Part model, mm, in its own coordinate system. Face numbers are marked on the shaded views. Round coordinates to 2 decimals unless told otherwise and drop trailing zeros. Write each loop counter-clockwise with the first axis right and the second up, starting at its lowest first coordinate (ties: lowest second). Pieces come first, ordered by that corner, then holes.
1) Saw through at B-B on x = 2. Write the cut outline in (y, z), and give its area (3 significant figures).
2) Flat gauge pins, fed straight in: pin 1 (1.5 mm diameter, centred on x = 0.5, z = 0, fed in from +Y); pin 2 (2 mm diameter, centred on x = 1, y = 23.5, fed in from -Z); pin 3 (3 mm diameter, centred on y = 21.5, z = -0.5, fed in from +X). Where does each tip first touch, or does it go through?
3) Saw through at D-D on y = 16.75. Write the cut outline in (x, z), and give its area (3 significant figures).
4) Saw through at C-C on z = 1.9. Write the cut outline in (x, y), and give its area (3 significant figures).
5) Pull direction Z, two halves, no side cores. Call the marked faces 1, 2 and 3: +Z half, -Z half, draft (parallel to the pull), parting line (faces both ways), or undercut.
6) Saw through at A-A on y = 25.5. Write the cut outline in (x, z), and give its area (3 significant figures).
7) Drill centre lines: L1, parallel to Y at x = -1.85, z = -1.4; L2, parallel to Z at x = -0.3, y = 26; L3, parallel to Z at x = 0.5, y = 26. Where is each one in solid material? Low to high.
```python
from build123d import *

# Parameters (mm, degrees)
SKETCH1_R                                           = 2.5
BOSS_EXTRUDE1_DEPTH                                 = 0.5
SKETCH2_R                                           = 2.25
BOSS_EXTRUDE2_DEPTH                                 = 27.7
CSK_FOR_M2_COUNTERSUNK_FLAT_HEAD_SCREW1_D           = 2.2
CSK_FOR_M2_COUNTERSUNK_FLAT_HEAD_SCREW1_DEPTH       = 9.339053319
CSK_FOR_M2_COUNTERSUNK_FLAT_HEAD_SCREW1_CSINK_D     = 3
CSK_FOR_M2_COUNTERSUNK_FLAT_HEAD_SCREW1_CSINK_ANGLE = 90
CSK_FOR_M2_COUNTERSUNK_FLAT_HEAD_SCREW1_TIP         = 0.660946681


with BuildPart() as part:
    # Sketch1 → Boss-Extrude1 (new body)
    with BuildSketch(Plane(origin=(0, 0, 0), x_dir=(1, 0, 0), z_dir=(0, 1, 0))):
        with Locations(Location((0, 0, 0), (0, 0, 270))):
            Circle(SKETCH1_R)
    extrude(amount=BOSS_EXTRUDE1_DEPTH)

    # Sketch2 → Boss-Extrude2 (add)
    with BuildSketch(Plane(origin=(0, 0.5, 0), x_dir=(1, 0, 0), z_dir=(0, 1, 0))):
        with Locations(Location((0, 0, 0), (0, 0, 270))):
            Circle(SKETCH2_R)
    extrude(amount=BOSS_EXTRUDE2_DEPTH)

    # CSK for M2 Countersunk Flat Head Screw1
    with Locations(Plane(origin=(0, 28.2, 0), x_dir=(1, 0, 0), z_dir=(0, 1, 0))):
        with Locations((0, 0)):
            CounterSinkHole(CSK_FOR_M2_COUNTERSUNK_FLAT_HEAD_SCREW1_D / 2, CSK_FOR_M2_COUNTERSUNK_FLAT_HEAD_SCREW1_CSINK_D / 2, depth=CSK_FOR_M2_COUNTERSUNK_FLAT_HEAD_SCREW1_DEPTH, counter_sink_angle=CSK_FOR_M2_COUNTERSUNK_FLAT_HEAD_SCREW1_CSINK_ANGLE)
            with Locations((0, 0, -(CSK_FOR_M2_COUNTERSUNK_FLAT_HEAD_SCREW1_DEPTH + CSK_FOR_M2_COUNTERSUNK_FLAT_HEAD_SCREW1_TIP / 2))):  # 118° drill point
                Cone(0, CSK_FOR_M2_COUNTERSUNK_FLAT_HEAD_SCREW1_D / 2, CSK_FOR_M2_COUNTERSUNK_FLAT_HEAD_SCREW1_TIP, mode=Mode.SUBTRACT)


solid = part.part
```
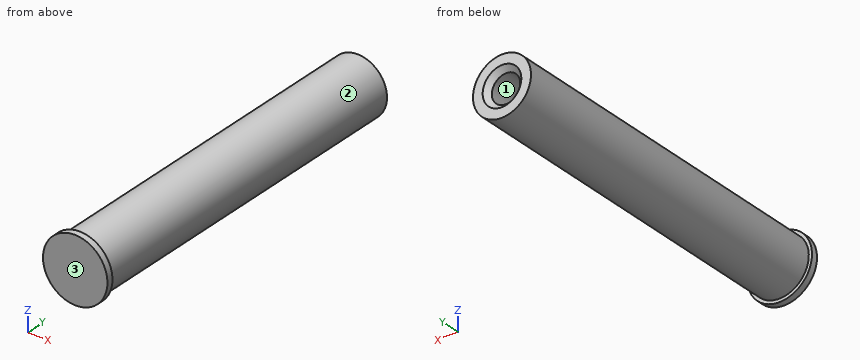
Completed:
1. outline: (0, -1.5) - (0.5, -1.5) - (0.5, -1.03) - (28.2, -1.03) - (28.2, 1.03) - (0.5, 1.03) - (0.5, 1.5) - (0, 1.5) - close
1. area: 58.6 mm2
2. pin 1: stops at y = 27.95
2. pin 2: stops at z = -2.25
2. pin 3: stops at x = 2.25
3. outline: circle Ø4.5 at (0, 0)
3. area: 15.9 mm2
4. outline: (-1.62, 0) - (1.62, 0) - (1.62, 0.5) - (1.21, 0.5) - (1.21, 28.2) - (-1.21, 28.2) - (-1.21, 0.5) - (-1.62, 0.5) - close
4. area: 68.4 mm2
5. face 1: undercut
5. face 2: parting line
5. face 3: draft
6. outline: circle Ø4.5 at (0, 0); hole circle Ø2.2 at (0, 0)
6. area: 12.1 mm2
7. L1: y = 0 to 0.5
7. L2: z = -2.23 to -1.06, 1.06 to 2.23
7. L3: z = -2.19 to -0.98, 0.98 to 2.19
